Job drawing, mm, ordinate dimensions from the low corner. One solid piece. Give positions to 0.01 mm unless a question says otherwise; leave off trailing zeros. Order: outer loops, then holes, each group sorted by start corner. A loop starts at its lowest first (then second) coordinate and runs counter-clockwise, first axis right, second up. Notation, with made-up numbers: M 27,74.5 L 60,74.5 A18 cw 60,79.5 Z; hole C 17,41 d11. An arc over 180 degrees is marked long. One line per question, with ' | ' between items.
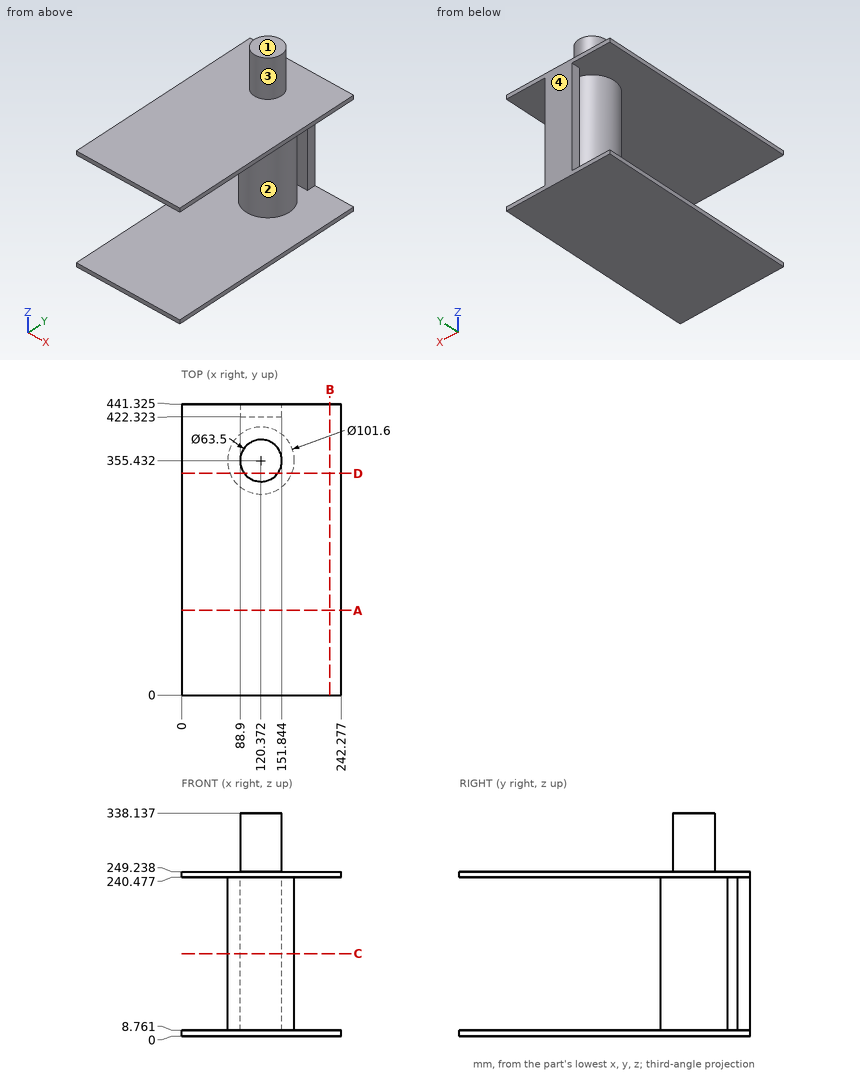
1. Slice it at C-C on z = 125. Give the cut face in (x, y) (1 decimal).
Worked out:
outline: C 120.4,355.4 d101.6; M 88.9,422.3 L 151.8,422.3 L 151.8,441.3 L 88.9,441.3 Z
2. Slice it at A-A on y = 128.5. Give the cut face in (x, z).
Worked out:
outline: M 0,0 L 242.28,0 L 242.28,8.76 L 0,8.76 Z; M 0,240.48 L 242.28,240.48 L 242.28,249.24 L 0,249.24 Z
3. Probe L1, parallel to Z at x = 143.5, y = 165; L2, parallel to Y at x = 142, z = 72 (1 decimal); L3, parallel to X at y = 358.5, z = 71.5 (1 decimal). List the from-to ranges inside material, lowest first. Write a range as from..to.
Worked out:
L1: z = 0..8.76, 240.48..249.24 | L2: y = 309.5..401.4, 422.3..441.3 | L3: x = 69.7..171.1
4. Slice it at D-D on y = 336. Give the cut face in (x, z) (1 decimal), then the cut area to 3 significant figures.
Worked out:
outline: M 0,0 L 242.3,0 L 242.3,8.8 L 167.3,8.8 L 167.3,240.5 L 242.3,240.5 L 242.3,249.2 L 145.5,249.2 L 145.5,338.1 L 95.3,338.1 L 95.3,249.2 L 0,249.2 L 0,240.5 L 73.4,240.5 L 73.4,8.8 L 0,8.8 Z | area: 30,500 mm2
5. Mould opens along Y. For the marked faces 1, 2, 3 and 4 say: released by +Y, released by -Y, zero draft, split by the parting line, or undercut.
Worked out:
face 1: zero draft | face 2: undercut | face 3: split by the parting line | face 4: released by +Y
6. Slice it at B-B on x = 225. Give the cut face in (y, z) (1 decimal), then the cut area to 3 significant figures.
Worked out:
outline: M 0,0 L 441.3,0 L 441.3,8.8 L 0,8.8 Z; M 0,240.5 L 441.3,240.5 L 441.3,249.2 L 0,249.2 Z | area: 7,730 mm2
7. Drop flat-ended pins along their axis: pin 1 (6 mm diameter, centred on x = 158.5, z = 219, fed in from +Y); pin 2 (2 mm diameter, centred on x = 27.5, y = 203, fed in from +Z); pin 3 (21 mm diameter, centred on y = 431.5, z = 140.5, fed in from +X). Give the stop position or say it passes through.
Worked out:
pin 1: stops at y = 392.13 | pin 2: stops at z = 249.24 | pin 3: stops at x = 151.84
